Check sheet for the modelled part. Datum: model origin and axes. Units: mm. A direction names the side the tool comes from. Give positions to 0.01 mm unless a question says otherwise; leave off trailing zeros. Loops run counter-clockwise (first coordinate to the right, second up) from the corner with the lowest first, then second, coordinate; pieces in that order, holes last. Notation, with made-up numbers: M 1.25,9 L 32.25,9 A20 cw 32.25,47 Z; hole C 87,44 d4. An arc over 180 degrees is marked long. Use one line per item in the form item = value.
from build123d import *

# Parameters (mm, degrees)
SKETCH1_W           = 220
SKETCH1_H           = 220
SKETCH1_R           = 5
SKETCH1_W_2         = 160
SKETCH1_H_2         = 160
BOSS_EXTRUDE1_DEPTH = 40
SKETCH4_W           = 30
SKETCH4_H           = 100
CUT_EXTRUDE1_DEPTH  = 286.657137142
SHELL1_START        = 10
SHELL1_DEPTH        = 20


# Read off the part's stored shape, not the designer's step: Shell1
with BuildPart() as part:
    # Sketch1 → Boss-Extrude1 (new body)
    with BuildSketch(Plane(origin=(0, 0, 0), x_dir=(1, 0, 0), z_dir=(0, 1, 0))):
        with Locations((90, 90)):
            Rectangle(SKETCH1_W, SKETCH1_H)
        with Locations(Location((0, 180, 0), (0, 0, 270))):
            Circle(SKETCH1_R, mode=Mode.SUBTRACT)
        with Locations(Location((180, 180, 0), (0, 0, 270))):
            Circle(SKETCH1_R, mode=Mode.SUBTRACT)
        with Locations(Location((180, 0, 0), (0, 0, 270))):
            Circle(SKETCH1_R, mode=Mode.SUBTRACT)
        with Locations(Location((0, 0, 0), (0, 0, 270))):
            Circle(SKETCH1_R, mode=Mode.SUBTRACT)
        with Locations((90, 90)):
            Rectangle(SKETCH1_W_2, SKETCH1_H_2, mode=Mode.SUBTRACT)
    extrude(amount=BOSS_EXTRUDE1_DEPTH)

    # Sketch4 → Cut-Extrude1 (cut, through all)
    with BuildSketch(Plane(origin=(0, 40, 0), x_dir=(1, 0, 0), z_dir=(0, 1, 0))):
        with Locations((185, 120)):
            Rectangle(SKETCH4_W, SKETCH4_H)
    extrude(amount=-CUT_EXTRUDE1_DEPTH, mode=Mode.SUBTRACT)

    # Shell1 outline → Shell1 (cut)
    with BuildSketch(Plane(origin=(0, 0, 0), x_dir=(1, 0, 0), z_dir=(0, 1, 0)).offset(SHELL1_START)):
        with BuildLine():
            Line((15, 180), (165, 180))
            ThreePointArc((165, 180), (180, 195), (195, 180))
            Line((195, 180), (200, 180))
            Line((200, 180), (200, 200))
            Line((200, 200), (-20, 200))
            Line((-20, 200), (-20, -20))
            Line((-20, -20), (200, -20))
            Line((200, -20), (200, 60))
            Line((200, 60), (180, 60))
            Line((180, 60), (180, 15))
            ThreePointArc((180, 15), (190.606601718, -10.606601718), (165, 0))
            Line((165, 0), (15, 0))
            ThreePointArc((15, 0), (-10.606601718, -10.606601718), (0, 15))
            Line((0, 15), (0, 165))
            ThreePointArc((0, 165), (-10.606601718, 190.606601718), (15, 180))
        make_face()
    extrude(amount=SHELL1_DEPTH, mode=Mode.SUBTRACT)


solid = part.part
1) Set-up check for faces 5 (the face through (104, 20, -170)), 6 (the face through (-10.25, 19.86, 10.95)), 7 (the face through (170, 20, -40)), 8 (the face through (197, 20, -180)): record each of +Z, -Z, +X, -X, +Y, -Y from which the full face is reachable in a straight line by a thin tool's end or side.
Evaluation:
face_5 = +X, +Y, -Y
face_6 = none
face_7 = +Y, -Y
face_8 = -Z, +X
2) Release check for a two-part mould opening along Z. For faces 1 (the face through (180, 20, -38)), 2 (the face through (-20, 5, -88)), 3 (the face through (88, 35, -200)), 4 (the face through (-10.95, 19.86, -190.25)) record: pulls with the +Z half, pulls with the -Z half, needs draft (parallel to the pull), parting line crosses it, or undercut.
Evaluation:
face_1 = undercut
face_2 = needs draft
face_3 = pulls with the -Z half
face_4 = undercut
3) Section check C-C (x = 51.5). Record the cut outline in (y, z), then the cut area to 3 significant figures.
Evaluation:
outline = M 0,-200 L 10,-200 L 10,-180 L 30,-180 L 30,-200 L 40,-200 L 40,-170 L 0,-170 Z; M 0,-10 L 40,-10 L 40,20 L 30,20 L 30,0 L 10,0 L 10,20 L 0,20 Z
area = 1,600 mm^2
4) Section check D-D (z = -122). Record the cut outline in (x, y), then the cut area to 3 significant figures.
Evaluation:
outline = M -20,0 L 10,0 L 10,40 L -20,40 L -20,30 L 0,30 L 0,10 L -20,10 Z
area = 800 mm^2
5) Section check B-B (y = 34.5). Record the cut outline in (x, z), then the cut area to 3 significant figures.
Evaluation:
outline = M -20,-200 L 200,-200 L 200,-170 L 10,-170 L 10,-10 L 170,-10 L 170,-70 L 200,-70 L 200,20 L -20,20 Z; hole C 0,-180 d10; hole C 0,0 d10; hole C 180,-180 d10; hole C 180,0 d10
area = 19,500 mm^2
6) Section check A-A (z = -54). Record the cut outline in (x, y).
Evaluation:
outline = M -20,0 L 10,0 L 10,40 L -20,40 L -20,30 L 0,30 L 0,10 L -20,10 Z; M 170,0 L 200,0 L 200,10 L 180,10 L 180,30 L 200,30 L 200,40 L 170,40 Z
7) Depth check by flat-ended pin: pin 1 Ø2 at (x, y) = (90, 28) entering from -Z; pin 2 Ø10 at (y, z) = (10, -147.5) entering from +X; pin 3 Ø9 at (x, y) = (191.5, 16.5) entering from -Z. Enter the tip coordinate at first touch or a pass-through.
Evaluation:
pin_1 = -180
pin_2 = 10
pin_3 = -193.27
8) Scan lines: line 1 (Z direction, x = 138, y = 26.5); line 2 (Y direction, x = 51.5, z = 6.5); line 3 (Z direction, x = 91.5, y = 38.5). Record each from-to range of solid material in increasing order.
Evaluation:
line_1 = -180 to -170, -10 to 0
line_2 = 0 to 10, 30 to 40
line_3 = -200 to -170, -10 to 20
